from build123d import *

# Parameters (mm, degrees)
SKETCH_1_W      = 88
SKETCH_1_H      = 88
EXTRUDE_1_DEPTH = 3
SKETCH_2_W      = 88
SKETCH_2_H      = 88
SKETCH_2_W_2    = 82
SKETCH_2_H_2    = 82
EXTRUDE_2_DEPTH = 7
SKETCH_3_R      = 1.5
SKETCH_3_W      = 8.5
SKETCH_3_H      = 17
SKETCH_3_R_2    = 1.2
SKETCH_3_W_2    = 17
SKETCH_3_H_2    = 8.5
SKETCH_3_W_3    = 6
SKETCH_3_H_3    = 6
EXTRUDE_3_DEPTH = 5
FILLET_1_R      = 5


with BuildPart() as part:
    # 草圖1 → 填料-伸長1 (new body)
    with BuildSketch(Plane(origin=(0, 0, 0), x_dir=(1, 0, 0), z_dir=(0, 1, 0))):
        with Locations((7.62917335, -5.98816568)):
            Rectangle(SKETCH_1_W, SKETCH_1_H)
    extrude(amount=EXTRUDE_1_DEPTH)

    # 草圖2 → 填料-伸長2 (add)
    with BuildSketch(Plane(origin=(0, 3, 0), x_dir=(1, 0, 0), z_dir=(0, 1, 0))):
        with Locations((7.62917335, -5.98816568)):
            Rectangle(SKETCH_2_W, SKETCH_2_H)
        with Locations((7.62917335, -5.98816568)):
            Rectangle(SKETCH_2_W_2, SKETCH_2_H_2, mode=Mode.SUBTRACT)
    extrude(amount=EXTRUDE_2_DEPTH)

    # 草圖3 → 填料-伸長3 (add)
    # profile 1 of 14: a face of its own
    with BuildSketch(Plane(origin=(0, 3, 0), x_dir=(1, 0, 0), z_dir=(0, 1, 0))):
        with Locations(Location((-13.37082665, 15.01183432, 0), (0, 0, 270))):
            Circle(SKETCH_3_R)
    # profile 2 of 14: a face of its own
    with BuildSketch(Plane(origin=(0, 3, 0), x_dir=(1, 0, 0), z_dir=(0, 1, 0))):
        with Locations(Location((6.62917335, 15.01183432, 0), (0, 0, 270))):
            Circle(SKETCH_3_R)
    # profile 3 of 14: a face of its own
    with BuildSketch(Plane(origin=(0, 3, 0), x_dir=(1, 0, 0), z_dir=(0, 1, 0))):
        with Locations(Location((26.62917335, 15.01183432, 0), (0, 0, 270))):
            Circle(SKETCH_3_R)
    # profile 4 of 14: a face of its own
    with BuildSketch(Plane(origin=(0, 3, 0), x_dir=(1, 0, 0), z_dir=(0, 1, 0))):
        with Locations(Location((6.62917335, -4.98816568, 0), (0, 0, 270))):
            Circle(SKETCH_3_R)
    # profile 5 of 14: a face of its own
    with BuildSketch(Plane(origin=(0, 3, 0), x_dir=(1, 0, 0), z_dir=(0, 1, 0))):
        with Locations(Location((26.62917335, -4.98816568, 0), (0, 0, 270))):
            Circle(SKETCH_3_R)
    # profile 6 of 14: a face of its own
    with BuildSketch(Plane(origin=(0, 3, 0), x_dir=(1, 0, 0), z_dir=(0, 1, 0))):
        with Locations(Location((26.62917335, -24.98816568, 0), (0, 0, 270))):
            Circle(SKETCH_3_R)
    # profile 7 of 14: a face of its own
    with BuildSketch(Plane(origin=(0, 3, 0), x_dir=(1, 0, 0), z_dir=(0, 1, 0))):
        with Locations(Location((-13.37082665, -4.98816568, 0), (0, 0, 270))):
            Circle(SKETCH_3_R)
    # profile 8 of 14: a face of its own
    with BuildSketch(Plane(origin=(0, 3, 0), x_dir=(1, 0, 0), z_dir=(0, 1, 0))):
        with Locations(Location((-13.37082665, -24.98816568, 0), (0, 0, 270))):
            Circle(SKETCH_3_R)
    # profile 9 of 14: a face of its own
    with BuildSketch(Plane(origin=(0, 3, 0), x_dir=(1, 0, 0), z_dir=(0, 1, 0))):
        with Locations(Location((6.62917335, -30.98816568, 0), (0, 0, 270))):
            Circle(SKETCH_3_R)
    # profile 10 of 14: a face of its own
    with BuildSketch(Plane(origin=(0, 3, 0), x_dir=(1, 0, 0), z_dir=(0, 1, 0))):
        with Locations((-29.12082665, 26.51183432)):
            Rectangle(SKETCH_3_W, SKETCH_3_H)
        with Locations(Location((-28.37082665, 22.01183432, 0), (0, 0, 270))):
            Circle(SKETCH_3_R_2, mode=Mode.SUBTRACT)
    # profile 11 of 14: a face of its own
    with BuildSketch(Plane(origin=(0, 3, 0), x_dir=(1, 0, 0), z_dir=(0, 1, 0))):
        with Locations((-29.12082665, -38.48816568)):
            Rectangle(SKETCH_3_W, SKETCH_3_H)
        with Locations(Location((-28.37082665, -33.98816568, 0), (0, 0, 270))):
            Circle(SKETCH_3_R_2, mode=Mode.SUBTRACT)
    # profile 12 of 14: a face of its own
    with BuildSketch(Plane(origin=(0, 3, 0), x_dir=(1, 0, 0), z_dir=(0, 1, 0))):
        with Locations((40.12917335, 30.76183432)):
            Rectangle(SKETCH_3_W_2, SKETCH_3_H_2)
        with Locations(Location((35.62917335, 30.01183432, 0), (0, 0, 270))):
            Circle(SKETCH_3_R_2, mode=Mode.SUBTRACT)
    # profile 13 of 14: a face of its own
    with BuildSketch(Plane(origin=(0, 3, 0), x_dir=(1, 0, 0), z_dir=(0, 1, 0))):
        with Locations((44.37917335, -42.73816568)):
            Rectangle(SKETCH_3_W, SKETCH_3_H_2)
    # profile 14 of 14: a face of its own
    with BuildSketch(Plane(origin=(0, 3, 0), x_dir=(1, 0, 0), z_dir=(0, 1, 0))):
        with Locations((39.12917335, -30.98816568)):
            Rectangle(SKETCH_3_W_3, SKETCH_3_H_3)
        with Locations(Location((39.12917335, -30.98816568, 0), (0, 0, 270))):
            Circle(SKETCH_3_R_2, mode=Mode.SUBTRACT)
    extrude(amount=EXTRUDE_3_DEPTH)

    # 圓角1
    fillet_1_edges = [part.edges().sort_by_distance(p)[0] for p in [
        (-24.87082665, 5.5, -18.01183432),
        (-24.87082665, 5.5, 29.98816568),
        (31.62917335, 5.5, -26.51183432),
        (-36.37082665, 5, -38.01183432),
        (51.62917335, 5, -38.01183432),
        (51.62917335, 5, 49.98816568),
        (-36.37082665, 5, 49.98816568),
        (40.12917335, 5.5, 38.48816568),
    ]]
    fillet(fillet_1_edges, radius=FILLET_1_R)


solid = part.part
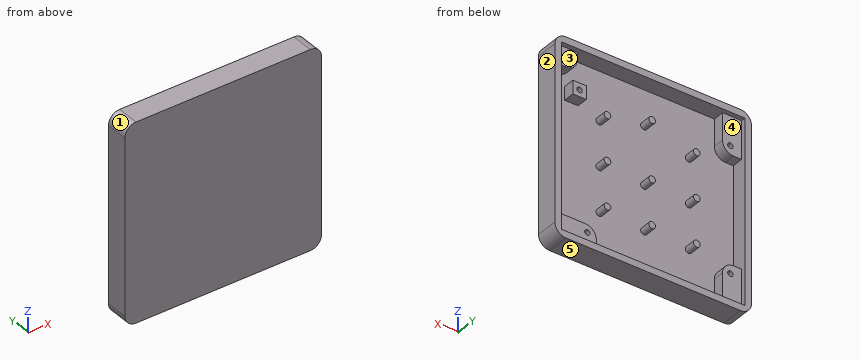
Could you check a few things on this model? Use its own coordinates, in mm. Face numbers are marked on the shaded views. A direction names the side the tool comes from. Coordinates: 2 decimals unless noted, no trailing zeros. Write each loop counter-clockwise with the first axis right and the second up, starting at its lowest first coordinate (ties: lowest second). Pieces come first, ordered by that corner, then holes. Notation, with made-up numbers: (36.5, 85) - (61.5, 85) arc R14 ccw to (61.5, 106) - close; hole circle Ø2 at (-31.5, 39.25). An arc over 180 degrees is marked (long way). Put each result on its own line as item: value. Start each with the question number.
Q1. I want a section at B-B on y = 9. Write out the boundary of the cut face in (x, z), plus the area to 3 significant figures.
Q2. I want a section at A-A on z = 2. Write out the boundary of the cut face in (x, y), plus the area to 3 significant figures.
Q3. Thinking about a two-plate mould opening in X: for the marked faces 1, 2 and 3, which applies, pulls with the +X half, pulls with the -X half, needs draft (parallel to the pull), parting line crosses it, or undercut?
Q4. Please list where these lines run through material, in increasing order: L1, parallel to X at y = 7.25, z = 12.5; L2, parallel to Z at x = -13, y = 6; L3, parallel to Z at x = -11.5, y = 5.5.
Q5. Which directions (+Z, -Z, +X, -X, +Y, -Y) give clear straight access to the entire face, cutting with the end or side of a thin tool? Please do the marked faces 4 and 5.
Q6. I'm going to push flat-ended pins straight in: P1, Ø0.7, axis at x = 35.5, z = -29.5, coming from the +Y side; P2, Ø1.5, axis at x = -13, z = -15, coming from the +Y side. Where does each tip first touch, or does it pass through?
Q7. I want a section at C-C on x = 14.5. Write out the boundary of the cut face in (y, z).
Checks:
1. outline: (-36.37, -33.01) arc R5 ccw to (-31.37, -38.01) - (46.63, -38.01) arc R5 ccw to (51.63, -33.01) - (51.63, 44.99) arc R5 ccw to (46.63, 49.99) - (-31.37, 49.99) arc R5 ccw to (-36.37, 44.99) - close; hole (-33.37, -35.01) - (48.63, -35.01) - (48.63, 46.99) - (-33.37, 46.99) - close
1. area: 999 mm²
2. outline: (-36.37, 0) - (51.63, 0) - (51.63, 10) - (48.63, 10) - (48.63, 3) - (-33.37, 3) - (-33.37, 10) - (-36.37, 10) - close
2. area: 306 mm²
3. face 1: pulls with the -X half
3. face 2: pulls with the +X half
3. face 3: undercut
4. L1: -36.37 to -33.37, 48.63 to 51.63
4. L2: -38.01 to -35.01, -16.47 to -13.56, 3.53 to 6.44, 23.53 to 26.44, 46.99 to 49.99
4. L3: -38.01 to -35.01, 46.99 to 49.99
5. face 4: +Y
5. face 5: -Z, +X, -X, +Y, -Y
6. P1: y = 3
6. P2: y = 8
7. outline: (0, -38.01) - (10, -38.01) - (10, -35.01) - (3, -35.01) - (3, 46.99) - (10, 46.99) - (10, 49.99) - (0, 49.99) - close
